```python
from build123d import *

# Parameters (mm, degrees)
BOSS_EXTRUDE1_DEPTH = 3.175
FILLET1_R           = 10


with BuildPart() as part:
    # Sketch1 → Boss-Extrude1 (new body)
    with BuildSketch(Plane.XY):
        Polygon((0, 20), (33.333333333, 20), (33.333333333, 23.175), (66.666666667, 23.175), (66.666666667, 20), (100, 20), (100, 0), (0, 0), align=None)
    extrude(amount=BOSS_EXTRUDE1_DEPTH)

    # Fillet1
    fillet1_edges = [part.edges().sort_by_distance(p)[0] for p in [
        (100, 0, 1.5875),
        (0, 0, 1.5875),
    ]]
    fillet(fillet1_edges, radius=FILLET1_R)


solid = part.part
```
Check sheet for the modelled part. Datum: model origin and axes. Units: mm. A direction names the side the tool comes from. Round coordinates to 2 decimals unless told otherwise and drop trailing zeros. Order: outer loops, then holes, each group sorted by start corner. A loop starts at its lowest first (then second) coordinate and runs counter-clockwise, first axis right, second up. Notation, with made-up numbers: (34.5, 5.25) -> (87.5, 5.25) arc R27 ccw to (87.5, 41.25) -> close; hole circle Ø8 at (39, -35.75). An arc over 180 degrees is marked (long way). One line per item, written item: value. Start each with the question number.
Q1. Gauge pin test, flat ends, axial feed: pin 1 Ø3 at (x, y) = (70, 15) entering from -Z; pin 2 Ø1.6 at (x, z) = (89.5, 2) entering from +Y; pin 3 Ø1.6 at (y, z) = (22, 1) entering from +X; pin 4 Ø1 at (y, z) = (4.5, 2.5) entering from -X. Record the tip position at first contact, or that the pin passes through.
Q2. Set-up check for faces 4 (the face through (16, 20, 2)), 5 (the face through (0, 15, 2)), 6 (the face through (66.667, 22, 2)): record each of +Z, -Z, +X, -X, +Y, -Y from which the full face is reachable in a straight line by a thin tool's end or side.
Q3. Thickness scan on line 1 (Y direction, x = 84, z = 3); line 2 (X direction, y = 1.25, z = 1.75); line 3 (X direction, y = 2, z = 0.7). Record the ranges inside material, lowest first.
Q4. Mould release check, pull along X, two halves, no side actions. Record for faces 1 (the face through (3.01, 2.85, 1.61)), 2 (the face through (100, 15, 2)), 3 (the face through (51, 12, 0)): pulls with the +X half, pulls with the -X half, needs draft (parallel to the pull), parting line crosses it, or undercut.
Q5. Cross-section at B-B (x = 77). Record the boundary of the cut face in (y, z) (3 decimals), and give its area (3 significant figures).
Q6. Cross-section at A-A (z = 1.1). Record the boundary of the cut face in (x, y) (3 decimals).
Q7. Cross-section at C-C (y = 5.75). Record the boundary of the cut face in (x, z) (3 decimals), and give its area (3 significant figures).
Completed:
1. pin 1: stops at z = 0
1. pin 2: stops at y = 20
1. pin 3: stops at x = 66.67
1. pin 4: stops at x = 1.34
2. face 4: +Z, -Z, -X, +Y
2. face 5: +Z, -Z, -X, +Y, -Y
2. face 6: +Z, -Z, +X, +Y
3. line 1: y = 0 to 20
3. line 2: x = 5.16 to 94.84
3. line 3: x = 4 to 96
4. face 1: pulls with the -X half
4. face 2: pulls with the +X half
4. face 3: needs draft
5. outline: (0, 0) -> (20, 0) -> (20, 3.175) -> (0, 3.175) -> close
5. area: 63.5 mm²
6. outline: (0, 10) arc R10 ccw to (10, 0) -> (90, 0) arc R10 ccw to (100, 10) -> (100, 20) -> (66.667, 20) -> (66.667, 23.175) -> (33.333, 23.175) -> (33.333, 20) -> (0, 20) -> close
7. outline: (0.948, 0) -> (99.052, 0) -> (99.052, 3.175) -> (0.948, 3.175) -> close
7. area: 311 mm²
